from build123d import *

# Parameters (mm, degrees)
F0_W     = 101.6
F0_H     = 25.4
F1_DEPTH = 63.5
F2_W     = 101.6
F2_H     = 36.316596
F3_DEPTH = 50.8
F4_W     = 51.353935
F4_H     = 40.734572
F5_DEPTH = 19.812


with BuildPart() as f1:
    # F0 (on Front) → F1 (new body)
    with BuildSketch(Plane.XZ):
        with Locations((24.13, -51.421492)):
            Rectangle(F0_W, F0_H)
    extrude(amount=F1_DEPTH)

    # F2 (on face) → F3 (join)
    with BuildSketch(Plane.XY.offset(-38.721492)):
        with Locations((24.13, -18.158298)):
            Rectangle(F2_W, F2_H)
    extrude(amount=F3_DEPTH)

    # F4 (on face) → F5 (cut)
    with BuildSketch(Plane.XZ.offset(36.316596)):
        with Locations((25.676967, -8.288778)):
            Rectangle(F4_W, F4_H)
    extrude(amount=-F5_DEPTH, mode=Mode.SUBTRACT)


solid = f1.part
The model under review builds one solid part; all positions refer to its coordinate system, in mm. A direction names the side the tool comes from. Round coordinates to 2 decimals unless told otherwise and drop trailing zeros. Loops run counter-clockwise (first coordinate to the right, second up) from the corner with the lowest first, then second, coordinate; pieces in that order, holes last. Notation, with made-up numbers: M -11.75,-10.75 L 21.25,-10.75 A15 cw 21.25,4.25 Z; hole C 0.25,11 d6. An arc over 180 degrees is marked long. Answer as CSV lines item,"result".
1. We need section D-D (x = -8.5). Give the boundary of the cut face in (y, z).
Outcome:
outline,"M -63.5,-64.12 L 0,-64.12 L 0,12.08 L -36.32,12.08 L -36.32,-38.72 L -63.5,-38.72 Z"
2. For faces 4 (the face through (23, -31, -64.121)), 5 (the face through (0, -27, -9)), 6 (the face through (23, -36.317, -31)), list the 3-axis set-ups (+Z, -Z, +X, -X, +Y, -Y) from which the entire face can be reached by the end or side of a thin tool; tool diameter is ignored.
Outcome:
face 4,"-Z, +X, -X, +Y, -Y"
face 5,"+Z, -Y"
face 6,"+Z, +X, -X, -Y"
3. To check wall thickness, follow L1, parallel to X at y = -31, z = -15; L2, parallel to Z at x = 27.5, y = -27; L3, parallel to Z at x = 27, y = -39. State the ranges of each line that lie inside material, in increasing order. Write a range as [from, to].
Outcome:
L1,"x = [-26.67, 0], [51.35, 74.93]"
L2,"z = [-64.12, -28.66]"
L3,"z = [-64.12, -38.72]"
4. We need section B-B (z = -10). Give the boundary of the cut face in (x, y), plus the area to 3 significant figures.
Outcome:
outline,"M -26.67,-36.32 L 0,-36.32 L 0,-16.5 L 51.35,-16.5 L 51.35,-36.32 L 74.93,-36.32 L 74.93,0 L -26.67,0 Z"
area,"2,670 mm2"
5. We need section C-C (y = -49). Give the boundary of the cut face in (x, z).
Outcome:
outline,"M -26.67,-64.12 L 74.93,-64.12 L 74.93,-38.72 L -26.67,-38.72 Z"
6. Insertion check: pin 1 Ø3 at (x, y) = (-3, -45) entering from +Z; pin 2 Ø15 at (x, z) = (34.5, -24) entering from -Y; pin 3 Ø10 at (x, y) = (14, -25.5) entering from +Z. Each pin has a flat end and moves straight along its axis. Give the tip position at first contact, or say it passes through.
Outcome:
pin 1,"stops at z = -38.72"
pin 2,"stops at y = -36.32"
pin 3,"stops at z = -28.66"
7. Draft analysis for pull direction X (two halves, no side actions). For faces 1 (the face through (25, -27, -28.656)), 2 (the face through (23, -14, 12.079)), 3 (the face through (-26.67, -25, -35)), state which applies: pulls with the +X half, pulls with the -X half, needs draft (parallel to the pull), parting line crosses it, or undercut.
Outcome:
face 1,"undercut"
face 2,"needs draft"
face 3,"pulls with the -X half"
8. We need section A-A (x = 8). Give the boundary of the cut face in (y, z), plus the area to 3 significant figures.
Outcome:
outline,"M -63.5,-64.12 L 0,-64.12 L 0,12.08 L -16.5,12.08 L -16.5,-28.66 L -36.32,-28.66 L -36.32,-38.72 L -63.5,-38.72 Z"
area,"2,650 mm2"
